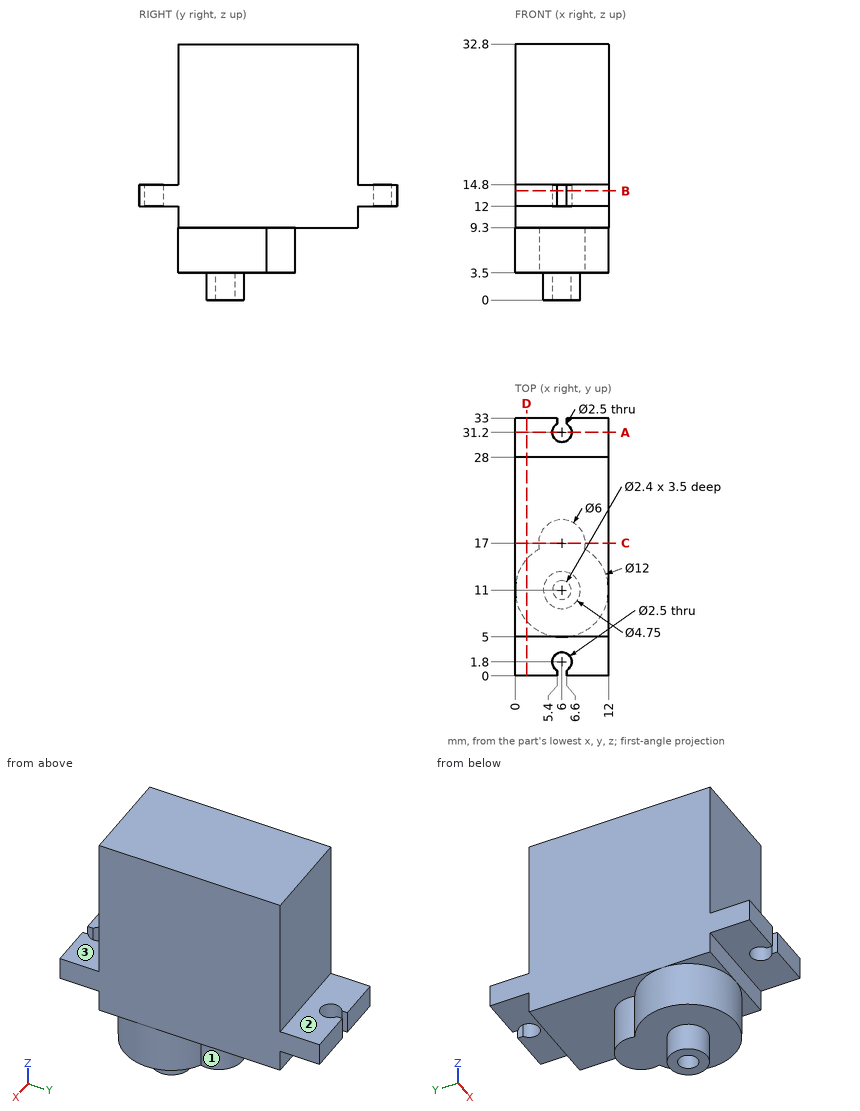
Design review of the part shown in the three views and the two pictorial views. Dimensions are in mm from the part's minimum x, y and z. A direction names the side the tool comes from. Give positions to 0.01 mm unless a question says otherwise; leave off trailing zeros. Loops run counter-clockwise (first coordinate to the right, second up) from the corner with the lowest first, then second, coordinate; pieces in that order, holes last. Notation, with made-up numbers: M 0,68.25 L 55,68.25 A28 ccw 55,107.25 Z; hole C 43.5,52.25 d11. An arc over 180 degrees is marked long. Answer as a JSON object with one key per item and string values. Group by question number.
Q1. Tool access review of the marked faces 1, 2 and 3: name each direction out of +Z, -Z, +X, -X, +Y, -Y from which nothing blocks a thin tool from reaching the whole face with its end or side.
Q2. Insertion check: P1, Ø3.5, axis at x = 7.5, y = 23, coming from the -Z side; P2, Ø3, axis at x = 7.5, z = 5, coming from the +Y side; P3, Ø1.4, axis at x = 8, z = 10.5, coming from the -Y side. Each pin has a flat end and moves straight along its axis. Give the tip position at first contact, or say it passes through.
Q3. Add section A-A on y = 31.2. Give the boundary of the cut face in (x, z), and give its area (3 significant figures).
Q4. Add section D-D on x = 1.5. Give the boundary of the cut face in (y, z), and give its area (3 significant figures).
Q5. Add section B-B on z = 14. Give the boundary of the cut face in (x, y).
Q6. For probe 1 along X at (y, z) = (11, 1) (3 decimals); probe 2 along X at (y, z) = (1.8, 13.4); probe 3 along Z at (x, y) = (9, 7), list the stretches that pass through material, from the lowest coordinate up. Write a range as [from, to].
Q7. Add section C-C on y = 17. Give the boundary of the cut face in (x, z).
Checked values:
{
 "1": {"face 1": "-Z", "face 2": "+Z, +X, -X, +Y", "face 3": "+Z, +X, -X, -Y"},
 "2": {"P1": "z = 9.3", "P2": "y = 20", "P3": "y = 5"},
 "3": {"outline": "M 0,12 L 4.75,12 L 4.75,14.8 L 0,14.8 Z; M 7.25,12 L 12,12 L 12,14.8 L 7.25,14.8 Z", "area": "26.6 mm²"},
 "4": {"outline": "M 0,12 L 5,12 L 5,9.3 L 7.03,9.3 L 7.03,3.5 L 14.97,3.5 L 14.97,9.3 L 28,9.3 L 28,12 L 33,12 L 33,14.8 L 28,14.8 L 28,32.8 L 5,32.8 L 5,14.8 L 0,14.8 Z", "area": "615 mm²"},
 "5": {"outline": "M 0,0 L 5.4,0 L 5.4,0.7 A1.25 cw long 6.6,0.7 L 6.6,0 L 12,0 L 12,33 L 6.6,33 L 6.6,32.3 A1.25 cw long 5.4,32.3 L 5.4,33 L 0,33 Z"},
 "6": {"probe 1": "[3.625, 4.8], [7.2, 8.375]", "probe 2": "[0, 4.75], [7.25, 12]", "probe 3": "[3.5, 32.8]"},
 "7": {"outline": "M 0,9.3 L 3,9.3 L 3,3.5 L 9,3.5 L 9,9.3 L 12,9.3 L 12,32.8 L 0,32.8 Z"}
}
